```python
from build123d import *

# Parameters (mm, degrees)
CUT_EXTRUDE_1_DEPTH      = 52.961524227
CUT_EXTRUDE_1_DEPTH_BACK = 52.961524227
SKETCH_2_R               = 10


with BuildPart() as part:
    # 草图1 → 旋转1 (revolve)
    with BuildSketch(Plane.XY):
        with BuildLine():
            Line((0, 30), (0, -30))
            ThreePointArc((0, -30), (30, 0), (0, 30))
        make_face()
    revolve(axis=Axis((0, 30, 0), (0, -1, 0)))

    # 草图2 → 切除-拉伸1 (cut, two sides: drawn at the far end of the back side and taken through both)
    with BuildSketch(Plane(origin=(0, 0, 0), x_dir=(1, 0, 0), z_dir=(0, 1, 0)).offset(-CUT_EXTRUDE_1_DEPTH_BACK)):
        Circle(SKETCH_2_R)
    extrude(amount=CUT_EXTRUDE_1_DEPTH + CUT_EXTRUDE_1_DEPTH_BACK, mode=Mode.SUBTRACT)

    # 草图4 → 旋转10 (revolve)
    with BuildSketch(Plane(origin=(0, 0, 0), x_dir=(0, 0, -1), z_dir=(1, 0, 0))):
        with BuildLine():
            Line((20.784609691, 20.784609691), (25.027250378, 16.541969004))
            Line((25.027250378, 16.541969004), (74.845263688, 57.946424516))
            ThreePointArc((74.845263688, 57.946424516), (79.16245845, 66.623512664), (75.660425587, 75.660425587))
            Line((75.660425587, 75.660425587), (20.784609691, 20.784609691))
        make_face()
    revolve(axis=Axis((0, 20.784609691, -20.784609691), (0, 0.7071067811865493, -0.7071067811865458)))


solid = part.part
```
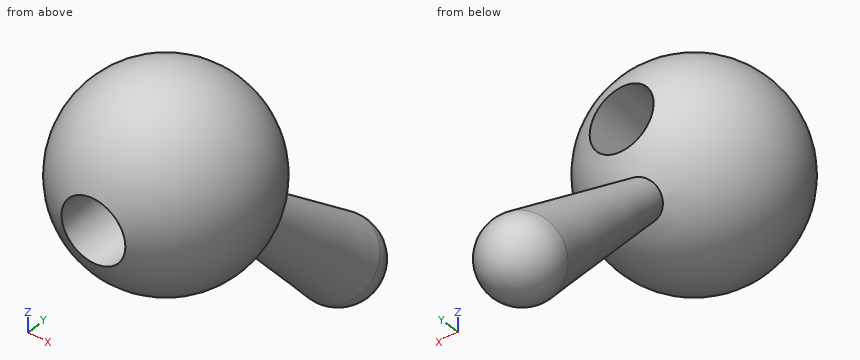
Check sheet for the modelled part. Datum: model origin and axes. Units: mm. Coordinates: 2 decimals unless noted, no trailing zeros. Loops run counter-clockwise (first coordinate to the right, second up) from the corner with the lowest first, then second, coordinate; pieces in that order, holes last.
1) Material ranges on probe 1 along Z at (x, y) = (0, -1); probe 2 along Z at (x, y) = (0, 8); probe 3 along Y at (x, z) = (-8.5, -70), recorded low to high.
2) Sectioned sample at D-D (y = -6.5). Record the boundary of the cut face in (x, z), and give its area (3 significant figures).
3) Sectioned sample at C-C (z = 18). Record the boundary of the cut face in (x, y).
4) Sectioned sample at B-B (x = 0). Record the boundary of the cut face in (y, z), and give its area (3 significant figures).
5) Gauge pin test, flat ends, axial feed: pin 1 (2 mm diameter, centred on x = -9, y = -15, fed in from +Z); pin 2 (3 mm diameter, centred on x = -9.5, z = -56, fed in from +Y); pin 3 (5 mm diameter, centred on y = -10.5, z = 6.5, fed in from +X). Record the tip position at first contact, or that the pin passes through.
6) Sectioned sample at A-A (z = 0). Record the boundary of the cut face in (x, y).
Check sheet entries:
1. probe 1: z = -29.98 to -10, 10 to 29.98
1. probe 2: z = -28.91 to -10, 10 to 28.91
1. probe 3: y = 58.67 to 75.16
2. outline: circle Ø58.57 at (0, 0); hole circle Ø20 at (0, 0)
2. area: 2,380 mm2
3. outline: circle Ø48 at (0, 0)
4. outline: (-28.28, -10) arc R30 ccw to (16.54, -25.03) - (57.95, -74.85) arc R12 ccw (long way) to (74.85, -57.95) - (25.03, -16.54) arc R30 ccw to (28.28, -10) - close; (-28.28, 10) - (28.28, 10) arc R30 ccw to start
4. area: 3,060 mm2
5. pin 1: stops at z = 25.06
5. pin 2: stops at y = 68.03
5. pin 3: stops at x = 28.34
6. outline: (-10, -28.28) - (-10, 28.28) arc R30 ccw to start; (10, -28.28) arc R30 ccw to (10, 28.28) - close
